Here's how the part is built. I have some questions about the finished solid (model axes, mm). A direction names the side the tool comes from. Round coordinates to 2 decimals unless told otherwise and drop trailing zeros. Order: outer loops, then holes, each group sorted by start corner. A loop starts at its lowest first (then second) coordinate and runs counter-clockwise, first axis right, second up. Notation, with made-up numbers: (-10, -5) -> (-6, -5) arc R11 cw to (-6, 1) -> close; hole circle Ø5 at (70.5, -12.5). An arc over 180 degrees is marked (long way). One line per item, written item: value.
```python
from build123d import *

# Parameters (mm, degrees)
F0_R          = 82.55
F0_R_2        = 76.2
F1_DEPTH      = 152.4
F3_DEPTH      = 82.551
F3_DEPTH_BACK = 82.551


with BuildPart() as f1:
    # F0 (on Front) → F1 (new body)
    with BuildSketch(Plane.XZ):
        Circle(F0_R)
        Circle(F0_R_2, mode=Mode.SUBTRACT)
    extrude(amount=F1_DEPTH)

    # F2 (on Top) → F3 (cut, two sides)
    with BuildSketch(Plane.XY) as f3_sk:
        with BuildLine():
            ThreePointArc((-10.656565316, 0), (-2.4931626729, -2.9712355724), (1.8504931473, -10.4946681436))
            Line((1.8504931473, -10.4946681436), (11.5856227827, -65.7053318564))
            ThreePointArc((11.5856227827, -65.7053318564), (15.9292786029, -73.2287644276), (24.0926812459, -76.2))
            Line((24.0926812459, -76.2), (82.55, -76.2))
            Line((82.55, -76.2), (82.55, 0))
            Line((82.55, 0), (-10.656565316, 0))
        make_face()
    extrude(amount=-F3_DEPTH, mode=Mode.SUBTRACT)
    extrude(f3_sk.sketch, amount=F3_DEPTH_BACK, mode=Mode.SUBTRACT)


solid = f1.part
```
Q1. I want a section at D-D on y = -32.5. Write out the boundary of the cut face in (x, z), then the cut area to 3 significant figures.
Answers:
outline: (5.73, -82.35) -> (5.73, -75.98) arc R76.2 cw (long way) to (5.73, 75.98) -> (5.73, 82.35) arc R82.55 ccw (long way) to start
area: 1,660 mm2
Q2. Which directions (+Z, -Z, +X, -X, +Y, -Y) give clear straight access to the entire face, cutting with the end or side of a thin tool? Please do faces 5 (the face through (77, -76.2, 0)), 6 (the face through (24, -152.4, -73)).
Answers:
face 5: +Z, -Z, +X, +Y
face 6: +Z, -Z, +X, -X, -Y
Q3. For P1, Ø10, axis at x = 10, y = -87, coming from the -Z side; P2, Ø4, axis at x = 14, y = -96.5, coming from the +Z side; P3, Ø6, axis at x = -20, y = -79, coming from the -Z side, each with a flat end and sliding along its axis, tell me the tip position at first contact or that it passes through.
Answers:
P1: z = -82.4
P2: z = 81.67
P3: z = -80.78
Q4. I want a section at B-B on x = -32. Write out the boundary of the cut face in (y, z).
Answers:
outline: (-152.4, -76.1) -> (0, -76.1) -> (0, -69.16) -> (-152.4, -69.16) -> close; (-152.4, 69.16) -> (0, 69.16) -> (0, 76.1) -> (-152.4, 76.1) -> close
Q5. I want a section at C-C on y = -128. Write out the boundary of the cut face in (x, z), then the cut area to 3 significant figures.
Answers:
outline: circle Ø165.1 at (0, 0); hole circle Ø152.4 at (0, 0)
area: 3,170 mm2
Q6. I need wall thicknesses on line 1 along X through (y, z) = (-98, 0); line 2 along X through (y, z) = (-63, 0). Which ranges of each line are inside material? Lowest first, please.
Answers:
line 1: -82.55 to -76.2, 76.2 to 82.55
line 2: -82.55 to -76.2
Q7. If we mould it in two halves opening along X, with no side actions, what happens to faces 1 (the face through (-76.126, -92.067, 3.35)), 2 (the face through (-82.47, -92.07, 3.63)), 3 (the face through (6.65, -37.71, 78.87)), 4 (the face through (-76.1, 0, 6.4))? For each: pulls with the +X half, pulls with the -X half, needs draft (parallel to the pull), parting line crosses it, or undercut.
Answers:
face 1: undercut
face 2: parting line crosses it
face 3: pulls with the +X half
face 4: needs draft
Q8. I want a section at A-A on z = 0. Write out the boundary of the cut face in (x, y), then the cut area to 3 significant figures.
Answers:
outline: (-82.55, -152.4) -> (-76.2, -152.4) -> (-76.2, 0) -> (-82.55, 0) -> close; (76.2, -152.4) -> (82.55, -152.4) -> (82.55, -76.2) -> (76.2, -76.2) -> close
area: 1,450 mm2
